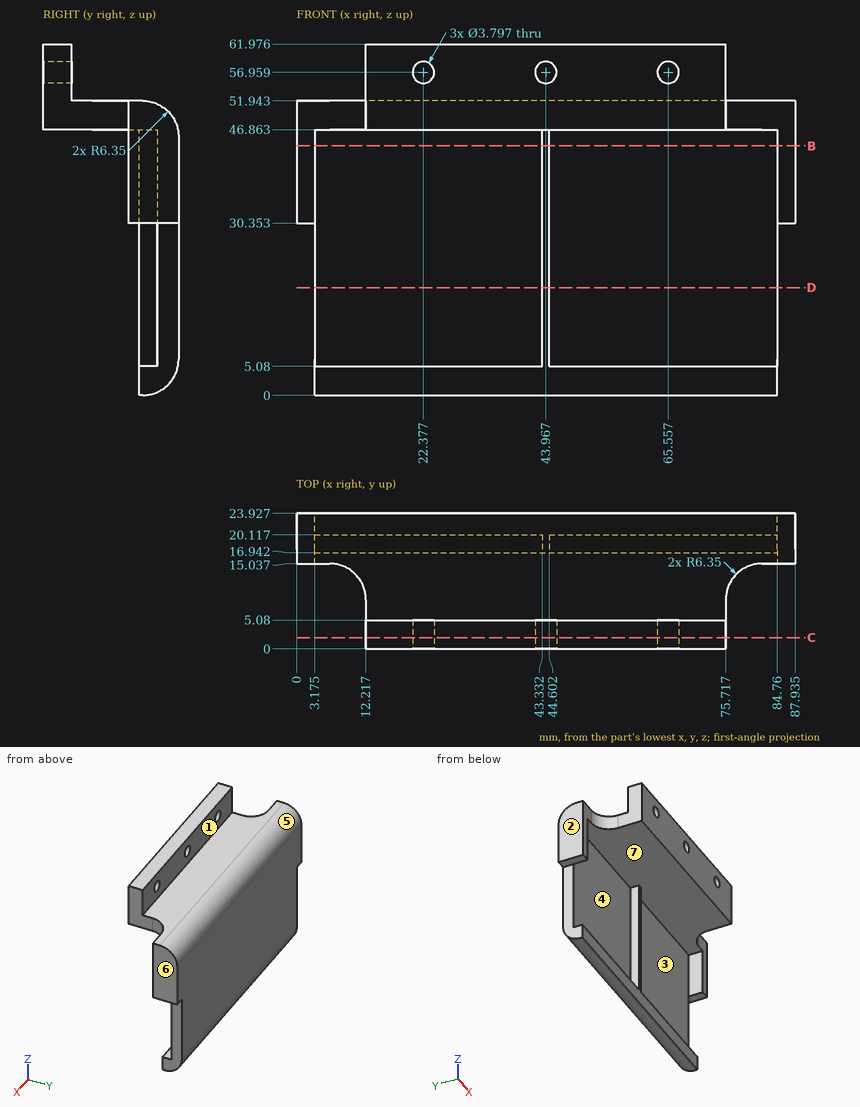
Here's the drawing with two shaded views (mm, measured from the low corner). I have some questions. A direction names the side the tool comes from. Give positions to 0.01 mm unless a question says otherwise; leave off trailing zeros. Loops run counter-clockwise (first coordinate to the right, second up) from the corner with the lowest first, then second, coordinate; pieces in that order, holes last. Notation, with made-up numbers: M 36.5,-24 L 40.5,-24 A29 cw 40.5,13 Z; hole C -16,30 d1. An arc over 180 degrees is marked long. One line per item, written item: value.
(1) Which directions (+Z, -Z, +X, -X, +Y, -Y) give clear straight access to the entire face, cutting with the end or side of a thin tool? Please do the marked faces 1, 2 and 3.
Returned:
face 1: +Z, +X, -X, +Y
face 2: +Z, -Z, -X, +Y, -Y
face 3: -Y
(2) I need wall thicknesses on line 1 (X direction, y = 18.25, z = 44) (1 decimal); line 2 (X direction, y = 16.75, z = 43) (1 decimal); line 3 (Y direction, x = 34, z = 42). Which ranges of each line are inside material? Lowest first, please.
Returned:
line 1: 0 to 3.2, 43.3 to 44.6, 84.8 to 87.9
line 2: 0 to 3.2, 84.8 to 87.9
line 3: 20.12 to 23.93
(3) We'd pull the mould along X, two halves only. Please class the marked faces 4, 5, 6 and 7: released by +X, released by -X, zero draft, split by the parting line, or undercut.
Returned:
face 4: undercut
face 5: zero draft
face 6: released by +X
face 7: undercut
(4) Suppose I cut it at B-B on z = 44. List the corners of the cut face in (x, y) for me (1 decimal).
Returned:
outline: M 0,15 L 3.2,15 L 3.2,20.1 L 43.3,20.1 L 43.3,16.9 L 44.6,16.9 L 44.6,20.1 L 84.8,20.1 L 84.8,15 L 87.9,15 L 87.9,23.9 L 0,23.9 Z
(5) Will these pins go through, and if not, where does the flat tip stop? pin 1 (2.5 mm diameter, centred on x = 58, y = 19, fed in from +Z); pin 2 (4.5 mm diameter, centred on x = 86.5, z = 40, fed in from -Y); pin 3 (6.5 mm diameter, centred on x = 4, z = 46.5, fed in from -Y).
Returned:
pin 1: z = 51.94
pin 2: y = 15.04
pin 3: y = 14.89
(6) Suppose I cut it at C-C on y = 2. List the corners of the cut face in (x, z) for me (1 decimal), plus the area to 3 significant figures.
Returned:
outline: M 12.2,46.9 L 75.7,46.9 L 75.7,62 L 12.2,62 Z; hole C 22.4,57 d3.8; hole C 44,57 d3.8; hole C 65.6,57 d3.8
area: 926 mm^2
(7) Suppose I cut it at D-D on z = 19. List the corners of the cut face in (x, y) for me (1 decimal).
Returned:
outline: M 3.2,20.1 L 43.3,20.1 L 43.3,16.9 L 44.6,16.9 L 44.6,20.1 L 84.8,20.1 L 84.8,23.9 L 3.2,23.9 Z
